from build123d import *

# Parameters (mm, degrees)
F0_W     = 25
F0_H     = 40
F1_DEPTH = 3
F3_D     = 2.15
F4_R     = 1
F6_D     = 6
F6_DEPTH = 4.05
F6_TIP   = 1.8025818571


with BuildPart() as f1:
    # F0 (on Top) → F1 (new body)
    with BuildSketch(Plane.XY):
        Rectangle(F0_W, F0_H)
    extrude(amount=F1_DEPTH)

    # F3 (through all)
    with Locations(Plane.XY.offset(3)):
        with Locations((0, 9.5), (0, -9.5), (8, 0), (-8, 0), (8, 16), (-8, 16), (-8, -16), (8, -16)):
            Hole(F3_D / 2)

    # F4
    f4_edges = [f1.edges().sort_by_distance(p)[0] for p in [
        (12.5, -20, 1.5),
        (-12.5, -20, 1.5),
        (12.5, 20, 1.5),
        (-12.5, 20, 1.5),
    ]]
    fillet(f4_edges, radius=F4_R)

    # F6
    with Locations(Plane.XY.offset(3)):
        with Locations((0, 0)):
            Hole(F6_D / 2, depth=F6_DEPTH)
            with Locations((0, 0, -(F6_DEPTH + F6_TIP / 2))):  # 118° drill point
                Cone(0, F6_D / 2, F6_TIP, mode=Mode.SUBTRACT)


solid = f1.part
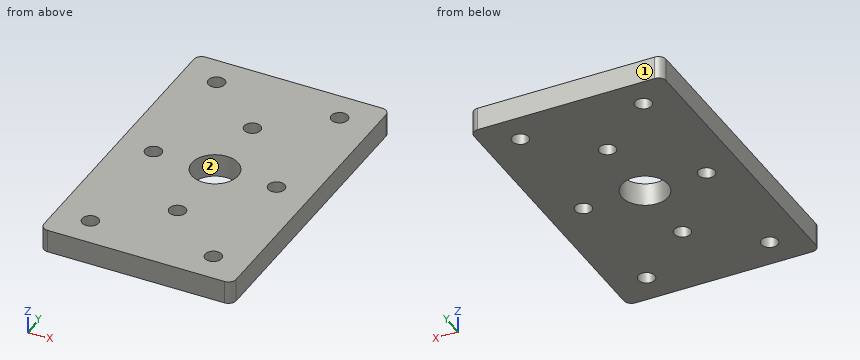
For this review, take the finished solid that the model builds, in its own axes (mm). Face numbers are marked on the shaded views. Round coordinates to 2 decimals unless told otherwise and drop trailing zeros. Write each loop counter-clockwise with the first axis right and the second up, starting at its lowest first coordinate (ties: lowest second). Pieces come first, ordered by that corner, then holes. Notation, with made-up numbers: (40, 11.25) -> (80, 11.25) arc R29 cw to (80, 33.25) -> close; hole circle Ø5 at (18, 25). An arc over 180 degrees is marked (long way). Put each result on its own line as item: value.
Q1. Consider section B-B on x = 0. State the section outline as (y, z) points (3 decimals).
Determined:
outline: (-20, 0) -> (-10.575, 0) -> (-10.575, 3) -> (-20, 3) -> close; (-8.425, 0) -> (-3, 0) -> (-3, 3) -> (-8.425, 3) -> close; (3, 0) -> (8.425, 0) -> (8.425, 3) -> (3, 3) -> close; (10.575, 0) -> (20, 0) -> (20, 3) -> (10.575, 3) -> close
Q2. Consider section D-D on y = 16. State the section outline as (x, z) points (3 decimals).
Determined:
outline: (-12.5, 0) -> (-9.075, 0) -> (-9.075, 3) -> (-12.5, 3) -> close; (-6.925, 0) -> (6.925, 0) -> (6.925, 3) -> (-6.925, 3) -> close; (9.075, 0) -> (12.5, 0) -> (12.5, 3) -> (9.075, 3) -> close
Q3. Clearance check with a flat-ended pin moving along its axis: pin 1 Ø1.9 at (x, y) = (-8, 16) entering from -Z. State where the tip first meets the part, or that it passes through.
Determined:
pin 1: passes through
Q4. The part is to be moulded in two halves that separate along X. For the marked faces 1 and 2, say which applies: released by +X, released by -X, zero draft, split by the parting line, or undercut.
Determined:
face 1: zero draft
face 2: undercut
Q5. Consider section A-A on y = -9.5. State the section outline as (x, z) points (3 decimals).
Determined:
outline: (-12.5, 0) -> (-1.075, 0) -> (-1.075, 3) -> (-12.5, 3) -> close; (1.075, 0) -> (12.5, 0) -> (12.5, 3) -> (1.075, 3) -> close
Q6. Consider section C-C on y = 0. State the section outline as (x, z) points (3 decimals).
Determined:
outline: (-12.5, 0) -> (-9.075, 0) -> (-9.075, 3) -> (-12.5, 3) -> close; (-6.925, 0) -> (-3, 0) -> (-3, 3) -> (-6.925, 3) -> close; (3, 0) -> (6.925, 0) -> (6.925, 3) -> (3, 3) -> close; (9.075, 0) -> (12.5, 0) -> (12.5, 3) -> (9.075, 3) -> close
Q7. To check wall thickness, follow L1, parallel to Y at x = 0, z = 1.45 (3 decimals); L2, parallel to Y at x = 8, z = 2.3 (3 decimals); L3, parallel to X at y = -15.5, z = 1.65. State the ranges of each line that lie inside material, in increasing order. Write a range as [from, to].
Determined:
L1: y = [-20, -10.575], [-8.425, -3], [3, 8.425], [10.575, 20]
L2: y = [-20, -17.075], [-14.925, -1.075], [1.075, 14.925], [17.075, 20]
L3: x = [-12.5, -8.95], [-7.05, 7.05], [8.95, 12.5]
